Autodesk Fusion 360 part; units mm, degrees
sketch "Sketch1" plane through (0, 0, 0) normal (0, 0, 1) x (1, 0, 0)
  line L0 (0, 0) -> (100, 0)
  line L1 (100, 0) -> (100, 100)
  line L2 (100, 100) -> (0, 100)
  line L3 (0, 100) -> (0, 0)
  line L4 (12.5, 87.5) -> (87.5, 87.5) construction
  line L5 (87.5, 87.5) -> (87.5, 12.5) construction
  line L6 (87.5, 12.5) -> (12.5, 12.5) construction
  line L7 (12.5, 12.5) -> (12.5, 87.5) construction
  line L8 (87.5, 50) -> (12.5, 50) construction
  line L9 (50, 87.5) -> (50, 12.5) construction
  circle A0 centre (12.5, 87.5) radius 2.25
  circle A1 centre (87.5, 87.5) radius 2.25
  circle A2 centre (12.5, 12.5) radius 2.25
  circle A3 centre (87.5, 12.5) radius 2.25
  line L10 (41.3, 45.8) -> (58.7, 45.8)
  line L11 (58.7, 45.8) -> (58.7, 54.2)
  line L12 (58.7, 54.2) -> (41.3, 54.2)
  line L13 (41.3, 54.2) -> (41.3, 45.8)
  dimension "d1" = 100
  dimension "d3" = 75
  dimension "d4" = 4.5
  dimension "d5" = 17.4
  dimension "d6" = 8.4
extrude "Extrude1" add sketch "Sketch1" along normal blind 10
sketch "Sketch2" plane through (0, 100, 0) normal (0, 1, 0) x (-1, 0, 0)
  line L0 (-100, 0) -> (0, 0)
  line L1 (0, 0) -> (0, 10)
  line L2 (0, 10) -> (-100, 10)
  line L3 (-100, 10) -> (-100, 0)
  circle A0 centre (-54, 5) radius 1.65
  circle A1 centre (-46, 5) radius 1.65
  line L4 (-50, 10) -> (-50, 0) construction
  line L5 (-54, 5) -> (-46, 5) construction
  dimension "d11" = 8
  dimension "d14" = 3.3
extrude "Extrude2" cut sketch "Sketch2" against normal up to surface (100 mm away) contours A0 | A1
sketch "Sketch3" plane through (0, 100, 0) normal (0, 1, 0) x (-1, 0, 0)
  circle A0 centre (-54, 5) radius 1.65
  circle A1 centre (-46, 5) radius 1.65
  line L0 (-100, 0) -> (0, 0)
  line L1 (0, 0) -> (0, 10)
  line L2 (0, 10) -> (-100, 10)
  line L3 (-100, 10) -> (-100, 0)
  circle A2 centre (-54, 5) radius 2.55
  circle A3 centre (-46, 5) radius 2.55
  dimension "d15" = 5.1
extrude "Extrude3" cut sketch "Sketch3" against normal blind 8 contours A2 | A3
sketch "Sketch4" plane through (0, 0, 0) normal (0, -1, 0) x (1, 0, 0)
  circle A0 centre (54, 5) radius 1.65
  circle A1 centre (46, 5) radius 1.65
  line L0 (0, 0) -> (100, 0)
  line L1 (100, 0) -> (100, 10)
  line L2 (100, 10) -> (0, 10)
  line L3 (0, 10) -> (0, 0)
  circle A2 centre (46, 5) radius 2.55
  circle A3 centre (54, 5) radius 2.55
  dimension "d18" = 5.1
extrude "Extrude4" cut sketch "Sketch4" against normal blind 8 contours A2 | A3
fillet "Fillet1" radius 0.8 4 edges at (48.3774, 100, 5.9221) (56.3774, 100, 5.9221) (51.6226, 0, 5.9221) (43.6226, 0, 5.9221)
fillet "Fillet3" radius 5 4 edges at (100, 0, 5) (0, 0, 5) (100, 100, 5) (0, 100, 5)
Model file for the job. Use its own axes, mm. A direction names the side the tool comes from. Round coordinates to 2 decimals unless told otherwise and drop trailing zeros. Write each loop counter-clockwise with the first axis right and the second up, starting at its lowest first coordinate (ties: lowest second). Pieces come first, ordered by that corner, then holes. Notation, with made-up numbers: M -40,38.25 L -28,38.25 A18 cw -28,62.25 Z; hole C -29.75,55.25 d11. An arc over 180 degrees is marked long. Put each result on its own line as item: value.
Item 1: Tool access for faces 4 (the cylindrical face through (99, 98, 5)), 5 (the flat face through (50, 54.2, 5)), 6 (the cylindrical face through (43.452, 4.35, 5.112)), 7 (the cylindrical face through (48.548, 95.65, 5.112)): list every direction of +Z, -Z, +X, -X, +Y, -Y with a clear straight run to the whole face (end or side of a thin tool).
Responses:
face 4: +Z, -Z, +X, +Y
face 5: +Z, -Z
face 6: -Y
face 7: +Y
Item 2: Cut at C-C (z = 5). State how many separate pieces and enclosed holes the cut face has, and give its area (3 significant figures).
Responses:
separate pieces: 4
enclosed holes: 4
area: 9,110 mm²
Item 3: Cut at B-B (x = 87.5). List the corners of the cut face in (y, z).
Responses:
outline: M 0,0 L 10.25,0 L 10.25,10 L 0,10 Z; M 14.75,0 L 85.25,0 L 85.25,10 L 14.75,10 Z; M 89.75,0 L 100,0 L 100,10 L 89.75,10 Z
Item 4: Mould opens along Z. For faces 1 (the flat face through (38, 51, 10)), 2 (the flat face through (50.6, 100, 3.8)), 3 (the cylindrical face through (55.65, 73.36, 5.07)) say: +Z half, -Z half, draft (parallel to the pull), parting line (faces both ways), or undercut.
Responses:
face 1: +Z half
face 2: draft
face 3: undercut
Item 5: Flat gauge pins, fed straight in: P1, Ø4, axis at x = 55, z = 4.5, coming from the -Y side; P2, Ø4.5, axis at x = 54, z = 5, coming from the -Y side; P3, Ø1.5, axis at x = 47, z = 5.5, coming from the +Y side. Where does each tip first touch, or does it go through?
Responses:
P1: y = 0.03
P2: y = 8
P3: y = 92
Item 6: Probe L1, parallel to Y at x = 87.5, z = 8; L2, parallel to X at y = 8.5, z = 4.25; L3, parallel to Z at x = 54, y = 68. List the from-to ranges inside material, lowest first. Write a range as from..to.
Responses:
L1: 0..10.25, 14.75..85.25, 89.75..100
L2: 0..44.53, 47.47..52.53, 55.47..100
L3: 0..3.35, 6.65..10
Item 7: Cut at A-A (y = 87.5). List the corners of the cut face in (x, z), and give its area (3 significant figures).
Responses:
outline: M 0,0 L 10.25,0 L 10.25,10 L 0,10 Z; M 14.75,0 L 85.25,0 L 85.25,10 L 14.75,10 Z; M 89.75,0 L 100,0 L 100,10 L 89.75,10 Z; hole C 46,5 d3.3; hole C 54,5 d3.3
area: 893 mm²
